Model file for the job. Use its own axes, mm. A direction names the side the tool comes from. Give positions to 0.01 mm unless a question says otherwise; leave off trailing zeros. Order: outer loops, then holes, each group sorted by start corner. A loop starts at its lowest first (then second) coordinate and runs counter-clockwise, first axis right, second up. Notation, with made-up numbers: (-11, 49) -> (26, 49) arc R22 cw to (26, 56) -> close; hole circle Ø9 at (-27, 16.5). An arc over 180 degrees is marked (long way). Use CSV: the item, a comma, the result in double quotes. Start each with the question number.
1. Cut at A-A on z = 1.25. List the corners of the cut face in (x, y) (3 decimals).
2. Cut at C-C on y = 10. List the corners of the cut face in (x, z), then the cut area to 3 significant figures.
3. Cut at D-D on z = 10. List the corners of the cut face in (x, y), then the cut area to 3 significant figures.
4. Cut at B-B on x = -34.5. List the corners of the cut face in (y, z).
5. Wall check: line 1 (X direction, y = 17.35, z = 5.9); line 2 (Y direction, x = -21, z = 8); line 3 (Y direction, x = -14.5, z = 0.75). Give the ranges that are in metal, low to high. Write a range as from..to.
6. 3-axis set-ups, long thin cutter, end or side, ignore diameter. For faces 1 (the flat face through (-17, 18, 6)), 2 (the flat face through (-44, 16, 6)), 3 (the flat face through (-44, 18, 6)), 4 (the flat face through (-14, 16, 6)), 5 (the flat face through (-19, 22, 11)): which of +Z, -Z, +X, -X, +Y, -Y reach the whole face in a straight line?
7. Pull direction Z, two halves, no side cores. Call faces 6 (the cylindrical face through (-25.48, 27.48, 7.12)), 7 (the flat face through (-12.996, 17, 6)), 8 (the cylindrical face through (-14.959, 17.014, 5.057)), 9 (the cylindrical face through (-43.695, 17.014, 5.856)): released by +Z, released by -Z, zero draft, split by the parting line, or undercut.
8. Drop flat-ended pins along their axis: pin 1 (1 mm diameter, centred on y = 5, z = 6, fed in from +X); pin 2 (1.2 mm diameter, centred on y = 20, z = 5, fed in from -X); pin 3 (2.5 mm diameter, centred on x = -16, z = 3.5, fed in from +Y). Give the stop position or say it passes through.
```python
from build123d import *

# Parameters (mm, degrees)
BOSS_EXTRU_1_DEPTH      = 11.8
ESQUISSE2_R             = 1
ENL_V_MAT_EXTRU_1_DEPTH = 11.8
ESQUISSE3_R             = 5.9
BOSS_EXTRU_2_DEPTH      = 4
ESQUISSE4_R             = 2
BOSS_EXTRU_3_DEPTH      = 3
ESQUISSE5_W             = 5
ESQUISSE5_H             = 4
BOSS_EXTRU_4_DEPTH      = 3
ESQUISSE6_W             = 3
ESQUISSE6_H             = 5
ENL_V_MAT_EXTRU_2_DEPTH = 10


with BuildPart() as part:
    # Esquisse1 → Boss.-Extru.1 (new body)
    with BuildSketch(Plane.XY):
        Polygon((-45.196459949, 18), (-40.196459949, 18), (-40.196459949, 22), (-17.996459949, 22), (-17.996459949, 18), (-12.996459949, 18), (-12.996459949, 16), (-17.996459949, 16), (-17.996459949, 0), (-40.196459949, 0), (-40.196459949, 16), (-45.196459949, 16), align=None)
    extrude(amount=BOSS_EXTRU_1_DEPTH)

    # Esquisse2 → Enlèv. mat.-Extru.1 (cut)
    with BuildSketch(Plane(origin=(0, 18, 0), x_dir=(1, 0, 0), z_dir=(0, 1, 0))):
        with Locations((-42.696459949, -5.9)):
            Circle(ESQUISSE2_R)
        with Locations((-15.496459949, -5.9)):
            Circle(ESQUISSE2_R)
    extrude(amount=-ENL_V_MAT_EXTRU_1_DEPTH, mode=Mode.SUBTRACT)

    # Esquisse3 → Boss.-Extru.2 (add)
    with BuildSketch(Plane(origin=(0, 22, 0), x_dir=(1, 0, 0), z_dir=(0, 1, 0))):
        with Locations((-23.896459949, -5.9)):
            Circle(ESQUISSE3_R)
    extrude(amount=BOSS_EXTRU_2_DEPTH)

    # Esquisse4 → Boss.-Extru.3 (add)
    with BuildSketch(Plane(origin=(0, 26, 0), x_dir=(1, 0, 0), z_dir=(0, 1, 0))):
        with Locations((-23.896459949, -5.9)):
            Circle(ESQUISSE4_R)
    extrude(amount=BOSS_EXTRU_3_DEPTH)

    # Esquisse5 → Boss.-Extru.4 (add)
    with BuildSketch(Plane(origin=(-17.996459949, 0, 0), x_dir=(0, 0, -1), z_dir=(1, 0, 0))):
        with Locations((-5.8, 5)):
            Rectangle(ESQUISSE5_W, ESQUISSE5_H)
    extrude(amount=BOSS_EXTRU_4_DEPTH)

    # Esquisse6 → Enlèv. mat.-Extru.2 (cut)
    with BuildSketch(Plane(origin=(0, 7, 0), x_dir=(1, 0, 0), z_dir=(0, 1, 0))):
        with Locations((-16.496459949, -5.8)):
            Rectangle(ESQUISSE6_W, ESQUISSE6_H)
    extrude(amount=-ENL_V_MAT_EXTRU_2_DEPTH, mode=Mode.SUBTRACT)


solid = part.part
```
Verdict:
1,outline,"(-45.196, 16) -> (-40.196, 16) -> (-40.196, 0) -> (-17.996, 0) -> (-17.996, 16) -> (-12.996, 16) -> (-12.996, 18) -> (-17.996, 18) -> (-17.996, 22) -> (-20.265, 22) -> (-20.265, 26) -> (-27.528, 26) -> (-27.528, 22) -> (-40.196, 22) -> (-40.196, 18) -> (-45.196, 18) -> close"
2,outline,"(-40.2, 0) -> (-18, 0) -> (-18, 11.8) -> (-40.2, 11.8) -> close"
2,area,"262 mm^2"
3,outline,"(-45.2, 16) -> (-40.2, 16) -> (-40.2, 0) -> (-18, 0) -> (-18, 16) -> (-13, 16) -> (-13, 18) -> (-18, 18) -> (-18, 22) -> (-19.65, 22) -> (-19.65, 26) -> (-28.14, 26) -> (-28.14, 22) -> (-40.2, 22) -> (-40.2, 18) -> (-45.2, 18) -> close"
3,area,"542 mm^2"
4,outline,"(0, 0) -> (22, 0) -> (22, 11.8) -> (0, 11.8) -> close"
5,line 1,"-45.2..-43.7, -41.7..-16.5, -14.5..-13"
5,line 2,"0..26"
5,line 3,"16..18"
6,face 1,"+Z, -Z, +X, +Y"
6,face 2,"+Z, -Z, -X, -Y"
6,face 3,"+Z, -Z, -X, +Y"
6,face 4,"+Z, -Z, +X, -Y"
6,face 5,"+Z, +X, +Y"
7,face 6,"split by the parting line"
7,face 7,"zero draft"
7,face 8,"undercut"
7,face 9,"undercut"
8,pin 1,"x = -18"
8,pin 2,"x = -40.2"
8,pin 3,"y = 18"
